Read the model definition and answer for the solid it produces. Units are mm, in the model's axes. Face numbers are marked on the shaded views. A direction names the side the tool comes from. Coordinates: 2 decimals unless noted, no trailing zeros. Order: outer loops, then holes, each group sorted by start corner. A loop starts at its lowest first (then second) coordinate and runs counter-clockwise, first axis right, second up. Notation, with made-up numbers: (66, -14.5) -> (110, -14.5) arc R23 cw to (110, 15.5) -> close; hole circle Ø11 at (-24, -23.75). An arc over 180 degrees is marked (long way). Answer in a Markdown table with one row per item.
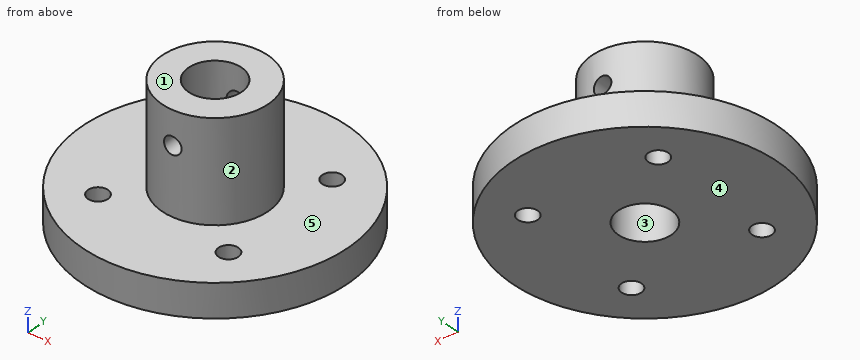
from build123d import *

# Parameters (mm, degrees)
SKETCH1_R               = 20
SKETCH1_R_2             = 4
SKETCH1_R_3             = 1.5
BOSS_EXTRUDE1_DEPTH     = 5
SKETCH2_R               = 8
SKETCH2_R_2             = 4
BOSS_EXTRUDE2_DEPTH     = 15
CUT_EXTRUDE1_DEPTH      = 35.641016151
CUT_EXTRUDE1_DEPTH_BACK = 35.641016151
SKETCH3_R               = 1.301925598


with BuildPart() as part:
    # Sketch1 → Boss-Extrude1 (new body)
    with BuildSketch(Plane.XY):
        Circle(SKETCH1_R)
        Circle(SKETCH1_R_2, mode=Mode.SUBTRACT)
        with Locations((-9.686203462, 9.686203462)):
            Circle(SKETCH1_R_3, mode=Mode.SUBTRACT)
        with Locations(Location((9.686203462, 9.686203462, 0), (0, 0, 180))):
            Circle(SKETCH1_R_3, mode=Mode.SUBTRACT)
        with Locations((9.686203462, -9.686203462)):
            Circle(SKETCH1_R_3, mode=Mode.SUBTRACT)
        with Locations(Location((-9.686203462, -9.686203462, 0), (0, 0, 180))):
            Circle(SKETCH1_R_3, mode=Mode.SUBTRACT)
    extrude(amount=BOSS_EXTRUDE1_DEPTH)

    # Sketch2 → Boss-Extrude2 (add)
    with BuildSketch(Plane.XY.offset(5)):
        Circle(SKETCH2_R)
        Circle(SKETCH2_R_2, mode=Mode.SUBTRACT)
    extrude(amount=BOSS_EXTRUDE2_DEPTH)

    # Sketch3 → Cut-Extrude1 (cut, two sides: drawn at the far end of the back side and taken through both)
    with BuildSketch(Plane(origin=(0, 0, 0), x_dir=(1, 0, 0), z_dir=(0, 1, 0)).offset(-CUT_EXTRUDE1_DEPTH_BACK)):
        with Locations(Location((0, -15, 0), (0, 0, 270))):
            Circle(SKETCH3_R)
    extrude(amount=CUT_EXTRUDE1_DEPTH + CUT_EXTRUDE1_DEPTH_BACK, mode=Mode.SUBTRACT)


solid = part.part
Q1. Given pin 1 (1 mm diameter, centred on y = 5, z = 14, fed in from +X); pin 2 (10 mm diameter, centred on y = -11, z = 10.5, fed in from +X); pin 3 (1.5 mm diameter, centred on y = 8, z = 17, fed in from +X), each flat-ended and moving along its own axis, determine where each tip first touches the part or whether it passes through.
Outcome:
| item | result |
|---|---|
| pin 1 | x = 6.61 |
| pin 2 | x = 5.29 |
| pin 3 | x = 3.38 |
Q2. The part is cut by section C-C (z = 11). Write down the section's boundary in (x, y), then the cut area to 3 significant figures.
Outcome:
| item | result |
|---|---|
| outline | circle Ø16 at (0, 0); hole circle Ø8 at (0, 0) |
| area | 151 mm² |
Q3. Consider line 1 (Y direction, x = -9.5, z = 2); line 2 (Y direction, x = 0, z = 7.25); line 3 (Z direction, x = -18, y = 6). Determine where each line is inside the solid, lowest interval first.
Outcome:
| item | result |
|---|---|
| line 1 | -17.6 to -11.17, -8.2 to 8.2, 11.17 to 17.6 |
| line 2 | -8 to -4, 4 to 8 |
| line 3 | 0 to 5 |
Q4. The part is cut by section D-D (z = 15). Write down the section's boundary in (x, y).
Outcome:
| item | result |
|---|---|
| outline | (-1.3, -7.89) -> (-1.3, -3.78) arc R4 cw to (-1.3, 3.78) -> (-1.3, 7.89) arc R8 ccw to start; (1.3, -7.89) arc R8 ccw to (1.3, 7.89) -> (1.3, 3.78) arc R4 cw to (1.3, -3.78) -> close |
Q5. For a pull along X with two mould halves and no side action, classify the marked faces 1, 2 and 3 as pulls with the +X half, pulls with the -X half, needs draft (parallel to the pull), parting line crosses it, or undercut.
Outcome:
| item | result |
|---|---|
| face 1 | needs draft |
| face 2 | parting line crosses it |
| face 3 | undercut |
Q6. For the marked faces 4 and 5, determine the directions among +Z, -Z, +X, -X, +Y, -Y from which every point of the face is accessible in a straight line to the end or side of a thin tool.
Outcome:
| item | result |
|---|---|
| face 4 | -Z, +X, -X, +Y, -Y |
| face 5 | +Z |
Q7. The part is cut by section A-A (x = 0). Write down the section's boundary in (y, z).
Outcome:
| item | result |
|---|---|
| outline | (-20, 0) -> (-4, 0) -> (-4, 13.7) -> (-8, 13.7) -> (-8, 5) -> (-20, 5) -> close; (-8, 16.3) -> (-4, 16.3) -> (-4, 20) -> (-8, 20) -> close; (4, 0) -> (20, 0) -> (20, 5) -> (8, 5) -> (8, 13.7) -> (4, 13.7) -> close; (4, 16.3) -> (8, 16.3) -> (8, 20) -> (4, 20) -> close |
Q8. The part is cut by section B-B (y = 0). Write down the section's boundary in (x, z), then the cut area to 3 significant figures.
Outcome:
| item | result |
|---|---|
| outline | (-20, 0) -> (-4, 0) -> (-4, 20) -> (-8, 20) -> (-8, 5) -> (-20, 5) -> close; (4, 0) -> (20, 0) -> (20, 5) -> (8, 5) -> (8, 20) -> (4, 20) -> close |
| area | 280 mm² |
